```python
from build123d import *

# Parameters (mm, degrees)
CYLINDER023_R     = 10
CYLINDER023_DEPTH = 10
CYLINDER022_R     = 14
CYLINDER022_DEPTH = 10
CYLINDER021_R     = 20
CYLINDER021_DEPTH = 3


with BuildPart() as cylinder007:
    # Cylinder023 → Cylinder023 (new body)
    with BuildSketch(Plane.XY):
        Circle(CYLINDER023_R)
    extrude(amount=CYLINDER023_DEPTH)


with BuildPart() as cylinder006:
    # Cylinder022 → Cylinder022 (new body)
    with BuildSketch(Plane.XY):
        Circle(CYLINDER022_R)
    extrude(amount=CYLINDER022_DEPTH)


with BuildPart() as cut032:
    # Cylinder021 → Cylinder021 (new body)
    with BuildSketch(Plane.XY):
        Circle(CYLINDER021_R)
    extrude(amount=CYLINDER021_DEPTH)

    # Fusion025: union Cylinder006
    add(cylinder006.part)

    # Cut032: cut Cylinder007
    add(cylinder007.part, mode=Mode.SUBTRACT)


with BuildPart() as cut032_1:
    # Cut032 placement: moved
    add(cut032.part.moved(Location((0, 0, -3))))


solid = cut032_1.part
```
Input: part model. Units: mm. Frame: model coordinates. A direction names the side the tool comes from. Coordinates: 2 decimals unless noted, no trailing zeros. Loops run counter-clockwise (first coordinate to the right, second up) from the corner with the lowest first, then second, coordinate; pieces in that order, holes last. Notation, with made-up numbers: M 65,47 L 78,47 A3 cw 78,52 Z; hole C 48,14.5 d2. An arc over 180 degrees is marked long. Use a Markdown table: item, result. Add a question column.
1) Section A-A, the plane y = 0. Return the cut outline in (x, z), plus the area to 3 significant figures.
2) Section C-C, the plane z = -1.25. Return the cut outline in (x, y), plus the area to 3 significant figures.
3) Section D-D, the plane x = 13. Return the cut outline in (y, z), plus the area to 3 significant figures.
4) Set-up query: faces 4 (the flat face through (-5, 9, -3)), 5 (the flat face through (-14, -4, 0)). Return all of +Z, -Z, +X, -X, +Y, -Y with unobstructed straight access to the full face (end or side cutting, diameter ignored); none if empty.
5) Draft query along X for faces 1 (the cylindrical face through (-4.336, -19.524, -1.521)), 2 (the flat face through (-3, 10, 7)), 3 (the cylindrical face through (-2.17, -9.76, 1.93)). Return one class per face: +X half, -X half, draft (parallel to the pull), parting line (faces both ways), or undercut.
6) Pin query (flat end, axial travel): P1, Ø3, axis at x = -8.5, z = 1, coming from the +Y side; P2, Ø6, axis at x = 0.5, z = 1.5, coming from the -Y side; P3, Ø6, axis at y = 11, z = 3.5, coming from the +X side. Return the tip coordinate at first contact, or that it passes through.
7) Line query: L1, parallel to Y at x = 0, z = 0.5; L2, parallel to Y at x = 0, z = -0.5; L3, parallel to Z at x = 14.5, y = -13. Output: solid intervals per line, ascending. Write a range as from..to.
Answer below:
| question | item | result |
|---|---|---|
| 1 | outline | M -20,-3 L -10,-3 L -10,7 L -14,7 L -14,0 L -20,0 Z; M 10,-3 L 20,-3 L 20,0 L 14,0 L 14,7 L 10,7 Z |
| 1 | area | 116 mm2 |
| 2 | outline | C 0,0 d40; hole C 0,0 d20 |
| 2 | area | 942 mm2 |
| 3 | outline | M -15.2,-3 L 15.2,-3 L 15.2,0 L 5.2,0 L 5.2,7 L -5.2,7 L -5.2,0 L -15.2,0 Z |
| 3 | area | 164 mm2 |
| 4 | face 4 | -Z, +X, -X, +Y, -Y |
| 4 | face 5 | +Z |
| 5 | face 1 | parting line |
| 5 | face 2 | draft |
| 5 | face 3 | undercut |
| 6 | P1 | y = 18.59 |
| 6 | P2 | y = -20 |
| 6 | P3 | x = 11.49 |
| 7 | L1 | -14..-10, 10..14 |
| 7 | L2 | -20..-10, 10..20 |
| 7 | L3 | -3..0 |
